```python
from build123d import *

# Parameters (mm, degrees)
SKETCH1_W                       = 96
SKETCH1_H                       = 96
BOSS_EXTRUDE1_DEPTH             = 8
SKETCH2_W                       = 92
SKETCH2_H                       = 92
COMPONENT_PLATFORM_DEPTH        = 6
CABLE_SLOTS_DEPTH               = 6
SKETCH4_R                       = 7.5
CENTER_MASS_CUT_DEPTH           = 6
INNER_CORNER_FILLETS_R          = 3
TAP_DRILL_FOR_M5X0_8_TAP2_D     = 4.2
TAP_DRILL_FOR_M5X0_8_TAP2_DEPTH = 2
TAP_DRILL_FOR_M2X0_4_TAP2_D     = 1.6
TAP_DRILL_FOR_M5X0_8_TAP1_D     = 4.2
TAP_DRILL_FOR_M5X0_8_TAP1_DEPTH = 2
CUT_EXTRUDE1_START              = -8
SKETCH28_OUTSIDE_W              = 125.2
SKETCH28_OUTSIDE_H              = 125.2
SKETCH28_OUTSIDE_W_2            = 95
SKETCH28_OUTSIDE_H_2            = 95
CUT_EXTRUDE1_DEPTH              = 8


with BuildPart() as part:
    # Sketch1 → Boss-Extrude1 (new body)
    with BuildSketch(Plane.XY):
        Rectangle(SKETCH1_W, SKETCH1_H)
    extrude(amount=BOSS_EXTRUDE1_DEPTH)

    # Sketch2 → Component Platform (cut)
    with BuildSketch(Plane.XY.offset(8)):
        Rectangle(SKETCH2_W, SKETCH2_H)
    extrude(amount=-COMPONENT_PLATFORM_DEPTH, mode=Mode.SUBTRACT)

    # Sketch3 → Cable Slots (cut, symmetric)
    with BuildSketch(Plane.XY.offset(2)):
        with BuildLine():
            Line((-40.878679656, -25.121320344), (-33.878679656, -18.121320344))
            ThreePointArc((-33.878679656, -18.121320344), (-33.228361402, -17.148050297), (-33, -16))
            Line((-33, -16), (-33, 16))
            ThreePointArc((-33, 16), (-33.228361402, 17.148050297), (-33.878679656, 18.121320344))
            Line((-33.878679656, 18.121320344), (-40.878679656, 25.121320344))
            ThreePointArc((-40.878679656, 25.121320344), (-41.851949703, 25.771638598), (-43, 26))
            Line((-43, 26), (-48, 26))
            Line((-48, 26), (-48, -26))
            Line((-48, -26), (-43, -26))
            ThreePointArc((-43, -26), (-41.851949703, -25.771638598), (-40.878679656, -25.121320344))
        make_face()
        with BuildLine():
            Line((48, -26), (48, 26))
            Line((48, 26), (43, 26))
            ThreePointArc((43, 26), (41.851949703, 25.771638598), (40.878679656, 25.121320344))
            Line((40.878679656, 25.121320344), (33.878679656, 18.121320344))
            ThreePointArc((33.878679656, 18.121320344), (33.228361402, 17.148050297), (33, 16))
            Line((33, 16), (33, -16))
            ThreePointArc((33, -16), (33.228361402, -17.148050297), (33.878679656, -18.121320344))
            Line((33.878679656, -18.121320344), (40.878679656, -25.121320344))
            ThreePointArc((40.878679656, -25.121320344), (41.851949703, -25.771638598), (43, -26))
            Line((43, -26), (48, -26))
        make_face()
    extrude(amount=CABLE_SLOTS_DEPTH, both=True, mode=Mode.SUBTRACT)

    # Sketch4 → Center Mass Cut (cut)
    with BuildSketch(Plane.XY.offset(2)):
        Circle(SKETCH4_R)
    extrude(amount=-CENTER_MASS_CUT_DEPTH, mode=Mode.SUBTRACT)

    # Inner Corner Fillets
    inner_corner_fillets_edges = [part.edges().sort_by_distance(p)[0] for p in [
        (-46, -46, 5),
        (-46, 46, 5),
        (46, 46, 5),
        (46, -46, 5),
    ]]
    fillet(inner_corner_fillets_edges, radius=INNER_CORNER_FILLETS_R)

    # Tap Drill for M5x0.8 Tap2
    with Locations(Plane(origin=(0, -48, 0), x_dir=(-1, 0, 0), z_dir=(0, -1, 0))):
        with Locations((35, -5), (-35, -5)):
            tap_drill_for_m5x0_8_tap2 = Hole(TAP_DRILL_FOR_M5X0_8_TAP2_D / 2, depth=TAP_DRILL_FOR_M5X0_8_TAP2_DEPTH)

    # Mirror2: Tap Drill for M5x0.8 Tap2 across plane
    add(tap_drill_for_m5x0_8_tap2.mirror(Plane(origin=(0, 0, 0), x_dir=(0, 0, 1), z_dir=(0, -1, 0))), mode=Mode.SUBTRACT)

    # Tap Drill for M2x0.4 Tap2 (through all)
    with Locations(Plane.XY.offset(2)):
        with Locations((-17.3, 34.575), (-17.3, 24.225), (-17.3, 14.975), (-17.3, 4.625), (17.3, 4.625), (17.3, 14.975), (17.3, 24.225), (17.3, 34.575), (17.3, -4.625), (17.3, -14.975), (17.3, -24.225), (17.3, -34.575), (-17.3, -4.625), (-17.3, -14.975), (-17.3, -24.225), (-17.3, -34.575)):
            Hole(TAP_DRILL_FOR_M2X0_4_TAP2_D / 2)

    # Tap Drill for M5x0.8 Tap1
    with Locations(Plane(origin=(48, 0, 0), x_dir=(0, 0, -1), z_dir=(1, 0, 0))):
        with Locations((-5, -35), (-5, 35)):
            tap_drill_for_m5x0_8_tap1 = Hole(TAP_DRILL_FOR_M5X0_8_TAP1_D / 2, depth=TAP_DRILL_FOR_M5X0_8_TAP1_DEPTH)

    # Mirror3: Tap Drill for M5x0.8 Tap1 across plane
    add(tap_drill_for_m5x0_8_tap1.mirror(Plane(origin=(0, 0, 0), x_dir=(0, 0, 1), z_dir=(1, 0, 0))), mode=Mode.SUBTRACT)

    # Sketch28 outside → Cut-Extrude1 (cut)
    with BuildSketch(Plane(origin=(0, 0, 0), x_dir=(-1, 0, 0), z_dir=(0, 0, -1)).offset(CUT_EXTRUDE1_START)):
        Rectangle(SKETCH28_OUTSIDE_W, SKETCH28_OUTSIDE_H)
        Rectangle(SKETCH28_OUTSIDE_W_2, SKETCH28_OUTSIDE_H_2, mode=Mode.SUBTRACT)
    extrude(amount=CUT_EXTRUDE1_DEPTH, mode=Mode.SUBTRACT)


solid = part.part
```
Design review of the part built by this model. Coordinates are the model's own, in mm. A direction names the side the tool comes from. Coordinates: 2 decimals unless noted, no trailing zeros. Loops run counter-clockwise (first coordinate to the right, second up) from the corner with the lowest first, then second, coordinate; pieces in that order, holes last.
Q1. We need section C-C on y = 20.5. State the section outline as (x, z) points, and give its area (3 significant figures).
Reported:
outline: (-36.26, 0) - (36.26, 0) - (36.26, 2) - (-36.26, 2) - close
area: 145 mm2
Q2. We need section B-B on x = -31. State the section outline as (y, z) points.
Reported:
outline: (-47.5, 0) - (47.5, 0) - (47.5, 8) - (46, 8) - (46, 2) - (-46, 2) - (-46, 8) - (-47.5, 8) - close
Q3. For pin 1 (3 mm diameter, centred on x = 5.5, y = 3.5, fed in from +Z); pin 2 (3.5 mm diameter, centred on y = 35, z = 5, fed in from +X); pin 3 (1.5 mm diameter, centred on y = -23, z = 2, fed in from -X); pin 4 (1.5 mm diameter, centred on y = 18.5, z = 1.5, fed in from -X), all flat-tipped, find the tip position at first contact; note any pin that passes through.
Reported:
pin 1: stops at z = 2
pin 2: passes through
pin 3: stops at x = -39.51
pin 4: stops at x = -35.01
Q4. We need section A-A on y = 0. State the section outline as (x, z) points.
Reported:
outline: (-33, 0) - (-7.5, 0) - (-7.5, 2) - (-33, 2) - close; (7.5, 0) - (33, 0) - (33, 2) - (7.5, 2) - close
Q5. To check wall thickness, follow line 1 (Y direction, x = 46.55, z = 5); line 2 (X direction, y = -38, z = 5.5). State the ranges of each line that lie inside material, in increasing order.
Reported:
line 1: y = -47.5 to -37.1, -32.9 to -26, 26 to 32.9, 37.1 to 47.5
line 2: x = -47.5 to -46, 46 to 47.5
Q6. Tool access review of faces 1 (the face through (46, -32.7, 5)), 2 (the face through (-46.3, -26, 3.1)), 3 (the face through (46.2, -26, 3.2)): name each direction out of +Z, -Z, +X, -X, +Y, -Y from which nothing blocks a thin tool from reaching the whole face with its end or side.
Reported:
face 1: +Z
face 2: +Z, -Z, -X
face 3: +Z, -Z, +X
Q7. The part is to be moulded in two halves that separate along Z. For faces 4 (the face through (-46.74, 32.95, 4.54)), 5 (the face through (10, 1, 0)), 6 (the face through (37.33, -21.57, 1.01)), say which applies: +Z half, -Z half, draft (parallel to the pull), parting line (faces both ways), or undercut.
Reported:
face 4: undercut
face 5: -Z half
face 6: draft
